Build history of the part. All positions in model axes, mm. A direction names the side the tool comes from. Coordinates: 2 decimals unless noted, no trailing zeros. Order: outer loops, then holes, each group sorted by start corner. A loop starts at its lowest first (then second) coordinate and runs counter-clockwise, first axis right, second up. Notation, with made-up numbers: M -21,36.25 L -13,36.25 A27 cw -13,66.25 Z; hole C -14.5,76 d8. An arc over 180 degrees is marked long. Write item = value, one per line. Start each with the question number.
Q1. 3-axis set-ups, long thin cutter, end or side, ignore diameter. For faces 5 (the face through (27.5, -0.7, 85.2)), 6 (the face through (-3.5, 45, 5)), 7 (the face through (9.83, 20.49, 55.07)): which of +Z, -Z, +X, -X, +Y, -Y reach the whole face in a straight line?
Q2. Pull direction Y, two halves, no side cores. Call faces 1 (the face through (-7.52, -47.32, 55.07)), 2 (the face through (27.5, -1, 30)), 3 (the face through (-6, 25, 55)), 4 (the face through (-36, -48.57, 55.07)): released by +Y, released by -Y, zero draft, split by the parting line, or undercut.
Q3. Band-saw the part on C-C on x = -7.5. Write the cut outline in (y, z).
Q4. Pin check, flat tips, straight feed: P1, Ø8, axis at x = -21, y = -8, coming from the +Z side; P2, Ø16.5, axis at x = -17.5, y = 2, coming from the -Z side; P3, Ø22, axis at y = -1, z = 26.5, coming from the -X side; P4, Ø24, axis at y = 12.5, z = 81.5, coming from the -X side. Stop position of each tip, or through.
Q5. Band-saw the part on B-B on z = 80. Write the cut outline in (x, y), plus the area to 3 significant figures.
Q6. Band-saw the part on A-A on y = -40. Write the cut outline in (x, z), plus the area to 3 significant figures.
Q7. Band-saw the part on D-D on x = 3. Write the cut outline in (y, z).
Q8. Drill centre lines: probe 1 along Z at (x, y) = (-20, 22); probe 2 along Y at (x, z) = (35.25, 80); probe 3 along Z at (x, y) = (33, 0). Where is each one in solid material? Low to high.
```python
from build123d import *

# Parameters (mm, degrees)
F1_DEPTH       = 10
F2_W           = 100
F2_H           = 90
F3_DEPTH       = 10
F5_W           = 100
F5_H           = 10
F6_DEPTH       = 65
F7_D           = 5.5
F7_CSINK_D     = 10
F7_CSINK_ANGLE = 90
F8_R           = 5
F9_R           = 10
F10_R          = 7.5
F11_DEPTH      = 10


with BuildPart() as f1:
    # F0 (on Top) → F1 (new body)
    with BuildSketch(Plane.XY):
        with BuildLine():
            Line((-11.5, 50), (-37.5, 50))
            Line((-37.5, 50), (-37.5, -50))
            Line((-37.5, -50), (37.5, -50))
            Line((37.5, -50), (37.5, 50))
            Line((37.5, 50), (-3.5, 50))
            Line((-3.5, 50), (-3.5, 40))
            ThreePointArc((-3.5, 40), (-7.5, 36), (-11.5, 40))
            Line((-11.5, 40), (-11.5, 50))
        make_face()
    extrude(amount=F1_DEPTH)

    # F2 (on face) → F3 (join)
    with BuildSketch(Plane.YZ.offset(37.5)):
        with Locations((0, 55)):
            Rectangle(F2_W, F2_H)
    extrude(amount=-F3_DEPTH)

    # F5 (on face) → F6 (join, through all)
    with BuildSketch(Plane(origin=(27.5, 0, 0), x_dir=(0, -1, 0), z_dir=(-1, 0, 0))):
        with Locations((0, 55)):
            Rectangle(F5_W, F5_H)
    extrude(amount=F6_DEPTH)

    # F7 (through all)
    with Locations(Plane(origin=(27.5, 0, 0), x_dir=(0, -1, 0), z_dir=(-1, 0, 0))):
        with Locations((0, 80)):
            CounterSinkHole(F7_D / 2, F7_CSINK_D / 2, counter_sink_angle=F7_CSINK_ANGLE)

    # F8
    f8_edges = [f1.edges().sort_by_distance(p)[0] for p in [
        (-37.5, 50, 5),
        (-37.5, -50, 5),
        (32.5, -50, 100),
        (32.5, 50, 100),
        (-37.5, 50, 55),
        (-37.5, -50, 55),
    ]]
    fillet(f8_edges, radius=F8_R)

    # F9
    f9_edges = [f1.edges().sort_by_distance(p)[0] for p in [
        (27.5, 0, 10),
        (27.5, 0, 60),
        (27.5, 0, 50),
    ]]
    fillet(f9_edges, radius=F9_R)

    # F10 (on face) → F11 (cut, through all)
    with BuildSketch(Plane.XY.offset(60)):
        with Locations((-5.8896257542, -40)):
            Circle(F10_R)
        with BuildLine():
            Line((-0.8896257542, 25), (-10.8896257542, 25))
            ThreePointArc((-10.8896257542, 25), (-21.496227472, 20.6066017178), (-25.8896257542, 10))
            Line((-25.8896257542, 10), (-25.8896257542, 0))
            ThreePointArc((-25.8896257542, 0), (-21.496227472, -10.6066017178), (-10.8896257542, -15))
            Line((-10.8896257542, -15), (-0.8896257542, -15))
            ThreePointArc((-0.8896257542, -15), (9.7169759636, -10.6066017178), (14.1103742458, 0))
            Line((14.1103742458, 0), (14.1103742458, 10))
            ThreePointArc((14.1103742458, 10), (9.7169759636, 20.6066017178), (-0.8896257542, 25))
        make_face()
    extrude(amount=-F11_DEPTH, mode=Mode.SUBTRACT)


solid = f1.part
```
Recorded:
q1.face_5 = +Z, -X, +Y, -Y
q1.face_6 = -Z, +Y
q1.face_7 = +Z
q2.face_1 = undercut
q2.face_2 = zero draft
q2.face_3 = undercut
q2.face_4 = released by -Y
q3.outline = M -50,0 L 36,0 L 36,10 L -50,10 Z; M -50,50 L -47.33,50 L -47.33,60 L -50,60 Z; M -32.67,50 L -15,50 L -15,60 L -32.67,60 Z; M 25,50 L 50,50 L 50,60 L 25,60 Z
q4.P1 = 60
q4.P2 = 0
q4.P3 = 26.43
q4.P4 = 27.49
q5.outline = M 27.5,-50 L 37.5,-50 L 37.5,-2.75 L 29.75,-2.75 L 27.5,-5 Z; M 27.5,5 L 29.75,2.75 L 37.5,2.75 L 37.5,50 L 27.5,50 Z
q5.area = 940 mm2
q6.outline = M -37.5,0 L 37.5,0 L 37.5,100 L 27.5,100 L 27.5,70 A10 cw 17.5,60 L 1.61,60 L 1.61,50 L 17.5,50 A10 cw 27.5,40 L 27.5,20 A10 cw 17.5,10 L -37.5,10 Z; M -37.5,50 L -13.39,50 L -13.39,60 L -37.5,60 Z
q6.area = 2,210 mm2
q7.outline = M -50,0 L 50,0 L 50,10 L -50,10 Z; M -50,50 L -14.49,50 L -14.49,60 L -50,60 Z; M 24.49,50 L 50,50 L 50,60 L 24.49,60 Z
q8.probe_1 = 0 to 10, 50 to 60
q8.probe_2 = -50 to -2.75, 2.75 to 50
q8.probe_3 = 0 to 77.25, 82.75 to 100
